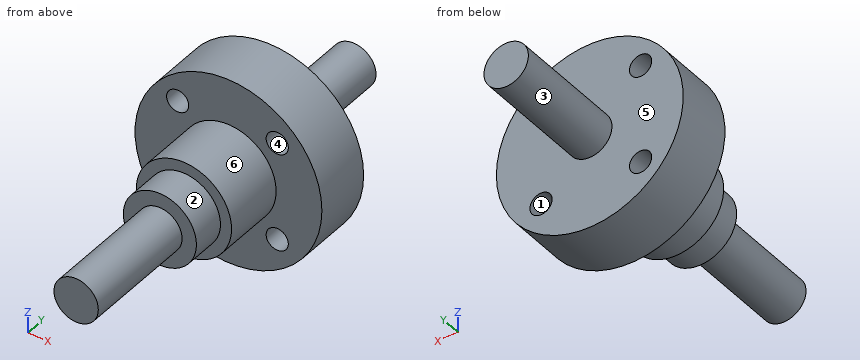
from build123d import *

# Parameters (mm, degrees)
F0_R          = 2.9972
F5_DEPTH      = 37.084
F5_DEPTH_BACK = 15.9766
F1_R          = 4.9403
F6_DEPTH      = 21.082
F2_R          = 6.4389
F7_DEPTH      = 16.4846
F3_R          = 12.6238
F8_DEPTH      = 7.9756
F9_D          = 2.9972


with BuildPart() as f5:
    # F0 (on Front) → F5 (new body, two sides)
    with BuildSketch(Plane.XZ) as f5_sk:
        Circle(F0_R)
    extrude(amount=F5_DEPTH)
    extrude(f5_sk.sketch, amount=-F5_DEPTH_BACK)

    # F1 (on Front) → F6 (join)
    with BuildSketch(Plane.XZ):
        Circle(F1_R)
    extrude(amount=F6_DEPTH)

    # F2 (on Front) → F7 (join)
    with BuildSketch(Plane.XZ):
        Circle(F2_R)
    extrude(amount=F7_DEPTH)

    # F3 (on Front) → F8 (join)
    with BuildSketch(Plane.XZ):
        Circle(F3_R)
    extrude(amount=F8_DEPTH)

    # F9 (through all)
    with Locations(Plane(origin=(0, 0, 0), x_dir=(1, 0, 0), z_dir=(0, 1, 0))):
        with Locations((-6.8628041832, -6.7065595315), (6.5900925825, -6.7065595315), (6.5900925825, 6.5454167448), (-6.8628041832, 6.5454167448)):
            Hole(F9_D / 2)


solid = f5.part
The model under review builds one solid part; all positions refer to its coordinate system, in mm. Face numbers are marked on the shaded views. A direction names the side the tool comes from. Coordinates: 2 decimals unless noted, no trailing zeros. Write each loop counter-clockwise with the first axis right and the second up, starting at its lowest first coordinate (ties: lowest second). Pieces come first, ordered by that corner, then holes. Notation, with made-up numbers: M -39.75,73.25 L 1.25,73.25 A12 cw 1.25,94.25 Z; hole C 59.5,82 d2. An arc over 180 degrees is marked long. Put each result on its own line as item: value.
1) Draft analysis for pull direction X (two halves, no side actions). For the marked faces 4, 5 and 6, state which applies: released by +X, released by -X, zero draft, split by the parting line, or undercut.
Computed:
face 4: undercut
face 5: zero draft
face 6: split by the parting line
2) Add section C-C on x = 0. Give the boundary of the cut face in (y, z).
Computed:
outline: M -37.08,-3 L -21.08,-3 L -21.08,-4.94 L -16.48,-4.94 L -16.48,-6.44 L -7.98,-6.44 L -7.98,-12.62 L 0,-12.62 L 0,-3 L 15.98,-3 L 15.98,3 L 0,3 L 0,12.62 L -7.98,12.62 L -7.98,6.44 L -16.48,6.44 L -16.48,4.94 L -21.08,4.94 L -21.08,3 L -37.08,3 Z
3) For the marked faces 1, 2 and 3, list the 3-axis set-ups (+Z, -Z, +X, -X, +Y, -Y) from which the entire face can be reached by the end or side of a thin tool; tool diameter is ignored.
Computed:
face 1: +Y, -Y
face 2: -Y
face 3: +Y
4) Wall thickness on probe 1 along Y at (x, z) = (-5.25, -9); probe 2 along Z at (x, y) = (-0.25, -19); probe 3 along Y at (x, z) = (6, -0.5): over which ranges is each line inside the solid? List them lowest first. Write a range as [from, to].
Computed:
probe 1: y = [-7.98, 0]
probe 2: z = [-4.93, 4.93]
probe 3: y = [-16.48, 0]
5) Add section D-D on y = -23.5. Give the boundary of the cut face in (x, z).
Computed:
outline: C 0,0 d5.99
6) Add section B-B on z = 0. Give the boundary of the cut face in (x, y), then the cut area to 3 significant figures.
Computed:
outline: M -12.62,-7.98 L -6.44,-7.98 L -6.44,-16.48 L -4.94,-16.48 L -4.94,-21.08 L -3,-21.08 L -3,-37.08 L 3,-37.08 L 3,-21.08 L 4.94,-21.08 L 4.94,-16.48 L 6.44,-16.48 L 6.44,-7.98 L 12.62,-7.98 L 12.62,0 L 3,0 L 3,15.98 L -3,15.98 L -3,0 L -12.62,0 Z
area: 548 mm2
7) Add section A-A on x = -7. Give the boundary of the cut face in (y, z), then the cut area to 3 significant figures.
Computed:
outline: M -7.98,-10.51 L 0,-10.51 L 0,-8.04 L -7.98,-8.04 Z; M -7.98,-5.05 L 0,-5.05 L 0,5.21 L -7.98,5.21 Z; M -7.98,8.2 L 0,8.2 L 0,10.51 L -7.98,10.51 Z
area: 120 mm2
8) Clearance check with flat-ended pins moving along their axes: pin 1 Ø6 at (y, z) = (10.5, 5.5) entering from +X; pin 2 Ø2 at (y, z) = (-5.5, -2) entering from +X; pin 3 Ø1 at (x, z) = (-5, 2.5) entering from -Y. State where each tip first meets the part, or that it passes through.
Computed:
pin 1: stops at x = 1.65
pin 2: stops at x = 12.58
pin 3: stops at y = -16.48
